from build123d import *

# Parameters (mm, degrees)
BOSS_EXTRUDE1_DEPTH = 355.6
CUT_EXTRUDE1_REACH  = 14.7
SKETCH3_R           = 9.525
CUT_EXTRUDE2_REACH  = 103.6
SKETCH4_R           = 6.35


with BuildPart() as part:
    # Sketch1 → Boss-Extrude1 (new body, symmetric)
    with BuildSketch(Plane.XY):
        with BuildLine():
            Line((0, 0), (0, 101.6))
            Line((0, 101.6), (3.18008, 101.6))
            ThreePointArc((3.18008, 101.6), (9.911679988, 98.811679988), (12.7, 92.08008))
            Line((12.7, 92.08008), (12.7, 22.225))
            ThreePointArc((12.7, 22.225), (15.489807909, 15.489807909), (22.225, 12.7))
            Line((22.225, 12.7), (92.08008, 12.7))
            ThreePointArc((92.08008, 12.7), (98.811679988, 9.911679988), (101.6, 3.18008))
            Line((101.6, 3.18008), (101.6, 0))
            Line((101.6, 0), (0, 0))
        make_face()
    extrude(amount=BOSS_EXTRUDE1_DEPTH, both=True)

    # Sketch3 → Cut-Extrude1 (cut, up to next)
    with BuildSketch(Plane(origin=(25.4, 12.7, 0), x_dir=(0, 0, -1), z_dir=(0, 1, 0)), mode=Mode.PRIVATE) as cut_extrude1_sk1:
        with Locations((330.2, -15.875)):
            Circle(SKETCH3_R)
    cut_extrude1_tool1 = extrude(cut_extrude1_sk1.sketch, amount=-CUT_EXTRUDE1_REACH, mode=Mode.PRIVATE) & part.part
    add(cut_extrude1_tool1.solids().sort_by_distance((41.275, 12.7, -330.2))[0], mode=Mode.SUBTRACT)
    # Sketch3 → Cut-Extrude1 (cut, up to next)
    with BuildSketch(Plane(origin=(25.4, 12.7, 0), x_dir=(0, 0, -1), z_dir=(0, 1, 0)), mode=Mode.PRIVATE) as cut_extrude1_sk2:
        with Locations((-330.2, -15.875)):
            Circle(SKETCH3_R)
    cut_extrude1_tool2 = extrude(cut_extrude1_sk2.sketch, amount=-CUT_EXTRUDE1_REACH, mode=Mode.PRIVATE) & part.part
    add(cut_extrude1_tool2.solids().sort_by_distance((41.275, 12.7, 330.2))[0], mode=Mode.SUBTRACT)
    # Sketch3 → Cut-Extrude1 (cut, up to next)
    with BuildSketch(Plane(origin=(25.4, 12.7, 0), x_dir=(0, 0, -1), z_dir=(0, 1, 0)), mode=Mode.PRIVATE) as cut_extrude1_sk3:
        with Locations((-330.2, -53.975)):
            Circle(SKETCH3_R)
    cut_extrude1_tool3 = extrude(cut_extrude1_sk3.sketch, amount=-CUT_EXTRUDE1_REACH, mode=Mode.PRIVATE) & part.part
    add(cut_extrude1_tool3.solids().sort_by_distance((79.375, 12.7, 330.2))[0], mode=Mode.SUBTRACT)
    # Sketch3 → Cut-Extrude1 (cut, up to next)
    with BuildSketch(Plane(origin=(25.4, 12.7, 0), x_dir=(0, 0, -1), z_dir=(0, 1, 0)), mode=Mode.PRIVATE) as cut_extrude1_sk4:
        with Locations((330.2, -53.975)):
            Circle(SKETCH3_R)
    cut_extrude1_tool4 = extrude(cut_extrude1_sk4.sketch, amount=-CUT_EXTRUDE1_REACH, mode=Mode.PRIVATE) & part.part
    add(cut_extrude1_tool4.solids().sort_by_distance((79.375, 12.7, -330.2))[0], mode=Mode.SUBTRACT)

    # Sketch4 → Cut-Extrude2 (cut, up to next)
    with BuildSketch(Plane.ZY, mode=Mode.PRIVATE) as cut_extrude2_sk1:
        with Locations((-52.4891, 25.4)):
            Circle(SKETCH4_R)
    cut_extrude2_tool1 = extrude(cut_extrude2_sk1.sketch, amount=-CUT_EXTRUDE2_REACH, mode=Mode.PRIVATE) & part.part
    add(cut_extrude2_tool1.solids().sort_by_distance((0, 25.4, -52.4891))[0], mode=Mode.SUBTRACT)
    # Sketch4 → Cut-Extrude2 (cut, up to next)
    with BuildSketch(Plane.ZY, mode=Mode.PRIVATE) as cut_extrude2_sk2:
        with Locations((52.4891, 25.4)):
            Circle(SKETCH4_R)
    cut_extrude2_tool2 = extrude(cut_extrude2_sk2.sketch, amount=-CUT_EXTRUDE2_REACH, mode=Mode.PRIVATE) & part.part
    add(cut_extrude2_tool2.solids().sort_by_distance((0, 25.4, 52.4891))[0], mode=Mode.SUBTRACT)


solid = part.part
Work out the finished part from the listing and answer in its coordinate system (mm). A direction names the side the tool comes from. Give positions to 0.01 mm unless a question says otherwise; leave off trailing zeros. Order: outer loops, then holes, each group sorted by start corner. A loop starts at its lowest first (then second) coordinate and runs counter-clockwise, first axis right, second up. Notation, with made-up numbers: (75, 36.25) -> (82, 36.25) arc R22 cw to (82, 54.25) -> close; hole circle Ø7 at (67.25, 76). An arc over 180 degrees is marked (long way). Answer as a JSON object with one key per item and string values. Group by question number.
1. A tool of negligible diameter and unlimited length cuts with its end or side. For faces 5 (the flat face through (12.7, 58, 5)), 6 (the cylindrical face through (40.856, 6.439, 339.716)), from which of +Z, -Z, +X, -X, +Y, -Y can it reach the whole face along a straight path? Write none if from no direction.
2. Section C-C on y = 73 is taken. Determine the outline of the cut face in (x, z).
3. The mould has two halves that part along Y. Classify faces 1 (the flat face through (57, 12.7, 5)), 2 (the flat face through (28, 10, 355.6)), 3 (the cylindrical face through (6.53, 22.968, 58.355)), 4 (the flat face through (52, 0, 5)): released by +Y, released by -Y, zero draft, split by the parting line, or undercut.
4. Consider line 1 along Z through (x, y) = (2, 25); line 2 along Z through (x, y) = (8, 25.4); line 3 along X through (y, z) = (5.5, 330.2). Determine where each line is inside the solid, lowest interval first. Write a range as [from, to].
5. Section A-A on z = -330.2 is taken. Determine the outline of the cut face in (x, y) (3 decimals).
6. Section B-B on z = 33 is taken. Determine the outline of the cut face in (x, y) (3 decimals).
7. Flat-ended cylindrical pins translate along their axes: pin 1 Ø10 at (y, z) = (22, 279) entering from +X; pin 2 Ø8 at (y, z) = (11.5, -81) entering from +X; pin 3 Ø12 at (y, z) = (36.5, -100) entering from -X; pin 4 Ø1.5 at (x, z) = (19.5, 11) entering from +Y. Find the tip coordinate at first contact, or state that the pin passes through.
Result sheet:
{
 "1": {"face 5": "+Z, -Z, +X, +Y", "face 6": "+Y, -Y"},
 "2": {"outline": "(0, -355.6) -> (12.7, -355.6) -> (12.7, 355.6) -> (0, 355.6) -> close"},
 "3": {"face 1": "released by +Y", "face 2": "zero draft", "face 3": "undercut", "face 4": "released by -Y"},
 "4": {"line 1": "z = [-355.6, -58.83], [-46.15, 46.15], [58.83, 355.6]", "line 2": "z = [-355.6, -58.84], [-46.14, 46.14], [58.84, 355.6]", "line 3": "x = [0, 31.75], [50.8, 69.85], [88.9, 101.31]"},
 "5": {"outline": "(0, 0) -> (31.75, 0) -> (31.75, 12.7) -> (22.225, 12.7) arc R9.525 cw to (12.7, 22.225) -> (12.7, 92.08) arc R9.52 ccw to (3.18, 101.6) -> (0, 101.6) -> close; (50.8, 0) -> (69.85, 0) -> (69.85, 12.7) -> (50.8, 12.7) -> close; (88.9, 0) -> (101.6, 0) -> (101.6, 3.18) arc R9.52 ccw to (92.08, 12.7) -> (88.9, 12.7) -> close"},
 "6": {"outline": "(0, 0) -> (101.6, 0) -> (101.6, 3.18) arc R9.52 ccw to (92.08, 12.7) -> (22.225, 12.7) arc R9.525 cw to (12.7, 22.225) -> (12.7, 92.08) arc R9.52 ccw to (3.18, 101.6) -> (0, 101.6) -> close"},
 "7": {"pin 1": "stops at x = 14.26", "pin 2": "stops at x = 100.56", "pin 3": "stops at x = 0", "pin 4": "stops at y = 13.36"}
}
